Design review of the part built by this model. Coordinates are the model's own, in mm. Coordinates: 2 decimals unless noted, no trailing zeros. Write each loop counter-clockwise with the first axis right and the second up, starting at its lowest first coordinate (ties: lowest second). Pieces come first, ordered by that corner, then holes.
Q1. To check wall thickness, follow probe 1 along X at (y, z) = (0, 44); probe 2 along Y at (x, z) = (4.75, 92.5); probe 3 along Y at (x, z) = (-4, 12.5). State the ranges of each line that lie inside material, in increasing order.
Q2. Clearance check with flat-ended pins moving along their axes: pin 1 Ø8 at (x, z) = (-3, 43.5) entering from +Y; pin 2 Ø0.5 at (x, z) = (0, 54.5) entering from -Y; pin 3 Ø2 at (x, y) = (-7.5, -1.5) entering from -Z. State where each tip first meets the part, or that it passes through.
Q3. Add section A-A, the plane y = 1.5. Give the boundary of the cut face in (x, z), plus the area to 3 significant figures.
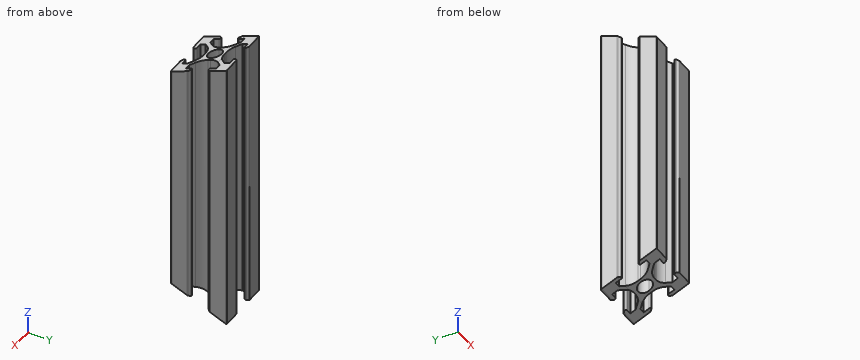
from build123d import *

# Parameters (mm, degrees)
RESSALTO_EXTRUS_O1_DEPTH = 100
PADR_OCIRCULAR1_COUNT    = 4
FILETE1_R                = 0.4
CUT_EXTRUDE1_DEPTH       = 103.46950766


with BuildPart() as part:
    # Esboço1 → Ressalto-extrusão1 (new body)
    with BuildSketch(Plane.XY):
        with BuildLine():
            ThreePointArc((-9.317157288, 3.217157288), (-9.187387948, 3.130448187), (-9.034314575, 3.1))
            Line((-9.034314575, 3.1), (-8.9, 3.1))
            ThreePointArc((-8.9, 3.1), (-8.617157288, 3.217157288), (-8.5, 3.5))
            Line((-8.5, 3.5), (-8.5, 5.5))
            Line((-8.5, 5.5), (-6.560660172, 5.5))
            Line((-6.560660172, 5.5), (-5.064466094, 4.003805922))
            ThreePointArc((-5.064466094, 4.003805922), (-3.980602337, 2.381689178), (-3.6, 0.468272016))
            Line((-3.6, 0.468272016), (-3.6, 0))
            Line((-3.6, 0), (-2.5, 0))
            ThreePointArc((-2.5, 0), (-1.767766953, 1.767766953), (0, 2.5))
            Line((0, 2.5), (0, 3.6))
            Line((0, 3.6), (-0.468272016, 3.6))
            ThreePointArc((-0.468272016, 3.6), (-2.381689178, 3.980602337), (-4.003805922, 5.064466094))
            Line((-4.003805922, 5.064466094), (-5.5, 6.560660172))
            Line((-5.5, 6.560660172), (-5.5, 8.5))
            Line((-5.5, 8.5), (-3.5, 8.5))
            ThreePointArc((-3.5, 8.5), (-3.217157288, 8.617157288), (-3.1, 8.9))
            Line((-3.1, 8.9), (-3.1, 9.034314575))
            ThreePointArc((-3.1, 9.034314575), (-3.130448187, 9.187387948), (-3.217157288, 9.317157288))
            Line((-3.217157288, 9.317157288), (-3.782842712, 9.882842712))
            ThreePointArc((-3.782842712, 9.882842712), (-3.912612052, 9.969551813), (-4.065685425, 10))
            Line((-4.065685425, 10), (-10, 10))
            Line((-10, 10), (-10, 4.065685425))
            ThreePointArc((-10, 4.065685425), (-9.969551813, 3.912612052), (-9.882842712, 3.782842712))
            Line((-9.882842712, 3.782842712), (-9.317157288, 3.217157288))
        make_face()
    ressalto_extrus_o1 = extrude(amount=RESSALTO_EXTRUS_O1_DEPTH)

    # PadrãoCircular1: Ressalto-extrusão1 ×4 about axis
    padr_ocircular1_axis = Axis((0, 0, 0), (0, 0, 1))
    for i in range(1, PADR_OCIRCULAR1_COUNT):
        add(ressalto_extrus_o1.rotate(padr_ocircular1_axis, i * 360 / PADR_OCIRCULAR1_COUNT))

    # Filete1
    filete1_edges = [part.edges().sort_by_distance(p)[0] for p in [
        (10, -10, 50),
        (10, 10, 50),
        (-10, 10, 50),
        (-10, -10, 50),
    ]]
    fillet(filete1_edges, radius=FILETE1_R)

    # Sketch1 → Cut-Extrude1 (cut, through all)
    with BuildSketch(Plane.ZY.offset(10)):
        Polygon((2.45807358, 4.065685425), (0, 4.065685425), (0, -10), (8.284271247, -10), align=None)
        Polygon((0.165685425, 9.6), (0, 9.6), (0, 4.065685425), (2.45807358, 4.065685425), align=None)
        Polygon((100, 9.6), (99.834314575, 9.6), (97.54192642, 4.065685425), (100, 4.065685425), align=None)
        Polygon((100, 4.065685425), (97.54192642, 4.065685425), (91.715728753, -10), (100, -10), (100, -9.6), align=None)
        Polygon((100, 10), (99.834314575, 9.6), (100, 9.6), align=None)
        Polygon((0.165685425, 9.6), (0, 10), (0, 9.6), align=None)
    extrude(amount=-CUT_EXTRUDE1_DEPTH, mode=Mode.SUBTRACT)


solid = part.part
Here are the results:
1. probe 1: x = -3.6 to -2.5, 2.5 to 3.6
1. probe 2: y = -5.81 to -3.66, 3.66 to 5.81, 8.5 to 10
1. probe 3: y = -9.99 to -8.5, -5.06 to -2.43, 2.43 to 5.06, 8.5 to 9.99
2. pin 1: stops at y = 10
2. pin 2: stops at y = -3.6
2. pin 3: passes through
3. outline: (-3.71, 3.52) - (-2, 3.52) - (-2, 96.48) - (-3.71, 96.48) - close; (2, 3.52) - (3.71, 3.52) - (3.71, 96.48) - (2, 96.48) - close
3. area: 317 mm2
